from build123d import *

# Parameters (mm, degrees)
SKETCH1_R           = 3.175
BOSS_EXTRUDE1_DEPTH = 1.3843


with BuildPart() as part:
    # Sketch1 → Boss-Extrude1 (new body, symmetric)
    with BuildSketch(Plane.XY):
        with BuildLine():
            Line((9.525, 11.270131987), (9.525, 25.4))
            ThreePointArc((9.525, 25.4), (0, 34.925), (-9.525, 25.4))
            Line((-9.525, 25.4), (-9.525, 11.270131987))
            ThreePointArc((-9.525, 11.270131987), (-8.829379111, 10.137441104), (-7.504545455, 10.245574533))
            ThreePointArc((-7.504545455, 10.245574533), (0, 12.7), (7.504545455, 10.245574533))
            ThreePointArc((7.504545455, 10.245574533), (8.829379111, 10.137441104), (9.525, 11.270131987))
        make_face()
        with Locations((0, 25.4)):
            Circle(SKETCH1_R, mode=Mode.SUBTRACT)
    extrude(amount=BOSS_EXTRUDE1_DEPTH, both=True)


solid = part.part
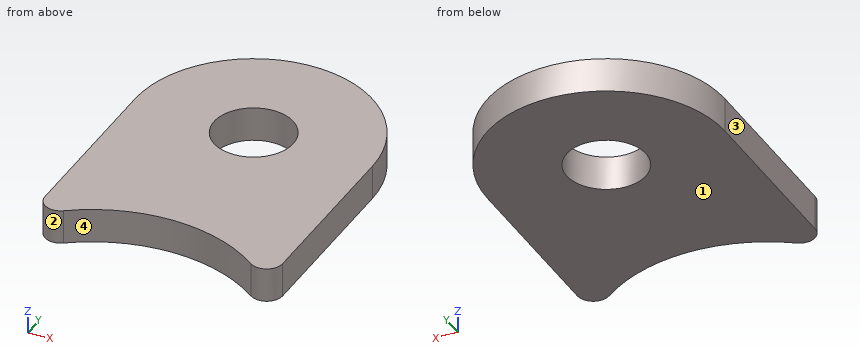
Build history of the part. All positions in model axes, mm. Face numbers are marked on the shaded views. Round coordinates to 2 decimals unless told otherwise and drop trailing zeros. Order: outer loops, then holes, each group sorted by start corner. A loop starts at its lowest first (then second) coordinate and runs counter-clockwise, first axis right, second up. Notation, with made-up numbers: M 2,51.25 L 27,51.25 A19 ccw 27,62.25 Z; hole C 12.25,-14.5 d4. An arc over 180 degrees is marked long. Use CSV: the item, a comma, the result in double quotes. Start each with the question number.
(1) Cut at C-C on y = 23.25. List the corners of the cut face in (x, z) (3 decimals), then the cut area to 3 significant figures.
(2) Flat gauge pin, fed straight in: P1, Ø1, axis at x = 4.5, z = -0.5, coming from the +Y side. Where does the tip first touch, or does it go through?
(3) Cut at A-A on z = 0.8. List the corners of the cut face in (x, y) (3 decimals), then the cut area to 3 significant figures.
(4) Cut at B-B on x = 0. List the corners of the cut face in (y, z) (3 decimals), then the cut area to 3 significant figures.
(5) Mould opens along X. For the marked faces 1, 2, 3 and 4 say: +X half, -X half, draft (parallel to the pull), parting line (faces both ways), or undercut.
(6) Drill centre lines: probe 1 along Y at (x, z) = (0, -0.2) (3 decimals); probe 2 along X at (y, z) = (27.25, -0.25); probe 3 along X at (y, z) = (25.75, -1). Where is each one in solid material? Low to high.
(7) Cut at D-D on y = 30. List the corners of the cut face in (x, z).
Findings:
1,outline,"M -9.525,-1.384 L -2.336,-1.384 L -2.336,1.384 L -9.525,1.384 Z; M 2.336,-1.384 L 9.525,-1.384 L 9.525,1.384 L 2.336,1.384 Z"
1,area,"39.8 mm^2"
2,P1,"stops at y = 34.04"
3,outline,"M -9.525,11.27 A1.27 ccw -7.505,10.246 A12.7 cw 7.505,10.246 A1.27 ccw 9.525,11.27 L 9.525,25.4 A9.525 ccw -9.525,25.4 Z; hole C 0,25.4 d6.35"
3,area,"375 mm^2"
4,outline,"M 12.7,-1.384 L 22.225,-1.384 L 22.225,1.384 L 12.7,1.384 Z; M 28.575,-1.384 L 34.925,-1.384 L 34.925,1.384 L 28.575,1.384 Z"
4,area,"44.0 mm^2"
5,face 1,"draft"
5,face 2,"undercut"
5,face 3,"-X half"
5,face 4,"undercut"
6,probe 1,"y = 12.7 to 22.225, 28.575 to 34.925"
6,probe 2,"x = -9.34 to -2.58, 2.58 to 9.34"
6,probe 3,"x = -9.52 to -3.16, 3.16 to 9.52"
7,outline,"M -8.34,-1.38 L 8.34,-1.38 L 8.34,1.38 L -8.34,1.38 Z"
